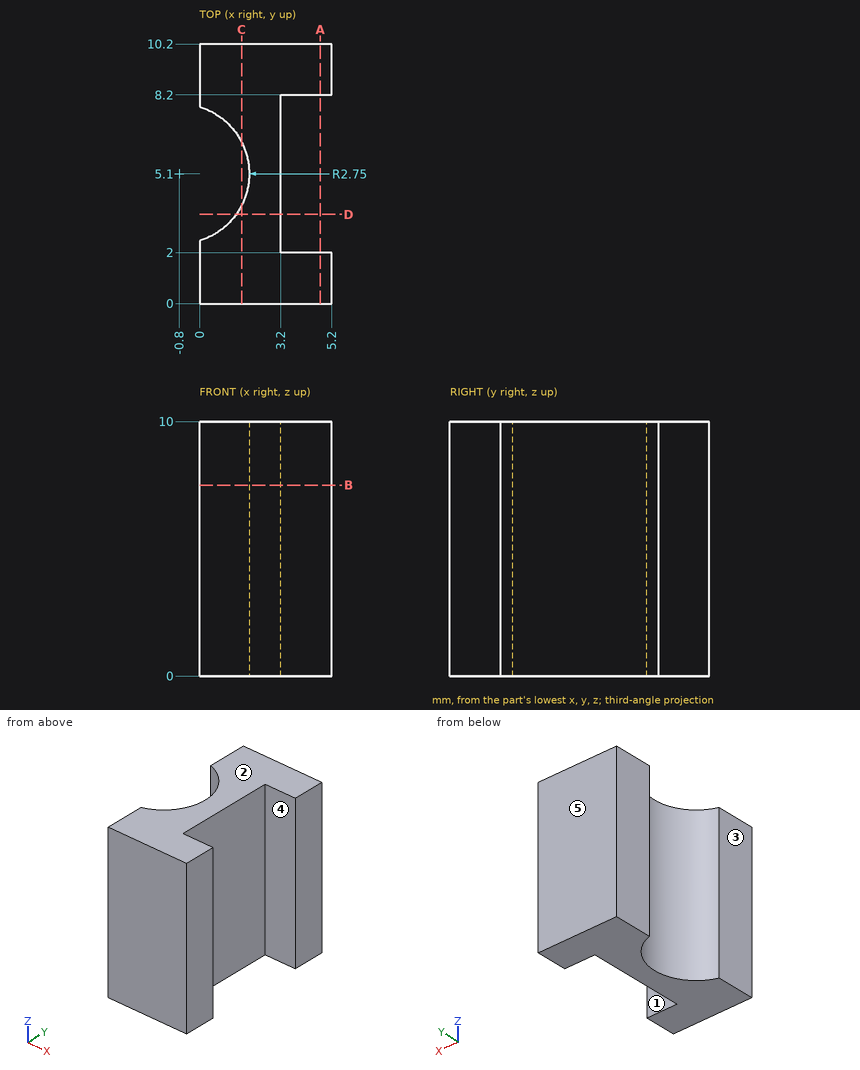
The drawing under review shows one solid part. Ordinate dimensions are in mm from its lowest x, y, z. A direction names the side the tool comes from. Coordinates: 2 decimals unless noted, no trailing zeros. Write each loop counter-clockwise with the first axis right and the second up, starting at its lowest first coordinate (ties: lowest second). Pieces come first, ordered by that corner, then holes. Notation, with made-up numbers: (50.25, 77) - (90.25, 77) arc R16 cw to (90.25, 107) - close; hole circle Ø8 at (86, 61). An arc over 180 degrees is marked (long way). Answer as CSV lines item,"result".
(1) Clearance check with flat-ended pins moving along their axes: pin 1 Ø1.9 at (y, z) = (4, 2.5) entering from +X; pin 2 Ø1 at (x, z) = (4.5, 3) entering from -Y; pin 3 Ø2 at (y, z) = (6, 3) entering from -X. State where each tip first meets the part, or that it passes through.
Data:
pin 1,"stops at x = 3.2"
pin 2,"stops at y = 0"
pin 3,"stops at x = 1.19"
(2) We need section D-D (y = 3.5). Give the boundary of the cut face in (x, z).
Data:
outline,"(1.44, 0) - (3.2, 0) - (3.2, 10) - (1.44, 10) - close"
(3) We need section C-C (x = 1.65). Give the boundary of the cut face in (y, z), plus the area to 3 significant figures.
Data:
outline,"(0, 0) - (3.85, 0) - (3.85, 10) - (0, 10) - close; (6.35, 0) - (10.2, 0) - (10.2, 10) - (6.35, 10) - close"
area,"77.0 mm2"
(4) Tool access review of the marked faces 1 and 2: name each direction out of +Z, -Z, +X, -X, +Y, -Y from which nothing blocks a thin tool from reaching the whole face with its end or side.
Data:
face 1,"+Z, -Z, +X"
face 2,"+Z, +X, -X, +Y, -Y"
(5) We need section A-A (x = 4.75). Give the boundary of the cut face in (y, z).
Data:
outline,"(0, 0) - (2, 0) - (2, 10) - (0, 10) - close; (8.2, 0) - (10.2, 0) - (10.2, 10) - (8.2, 10) - close"
(6) We need section B-B (z = 7.5). Give the boundary of the cut face in (x, y), plus the area to 3 significant figures.
Data:
outline,"(0, 0) - (5.2, 0) - (5.2, 2) - (3.2, 2) - (3.2, 8.2) - (5.2, 8.2) - (5.2, 10.2) - (0, 10.2) - (0, 7.73) arc R2.75 cw to (0, 2.47) - close"
area,"33.1 mm2"
(7) Mouldability with a two-part tool opening along Y and no side actions: class the marked faces 3, 4 and 5 as pulls with the +Y half, pulls with the -Y half, needs draft (parallel to the pull), parting line crosses it, or undercut.
Data:
face 3,"needs draft"
face 4,"undercut"
face 5,"pulls with the +Y half"
(8) For line 1 along Y through (x, z) = (4.4, 1); line 2 along Y through (x, z) = (1.15, 6.75); line 3 along X through (y, z) = (5, 6.5), list the stretches that pass through material, from the lowest coordinate up. Write a range as [from, to].
Data:
line 1,"y = [0, 2], [8.2, 10.2]"
line 2,"y = [0, 3.16], [7.04, 10.2]"
line 3,"x = [1.95, 3.2]"
